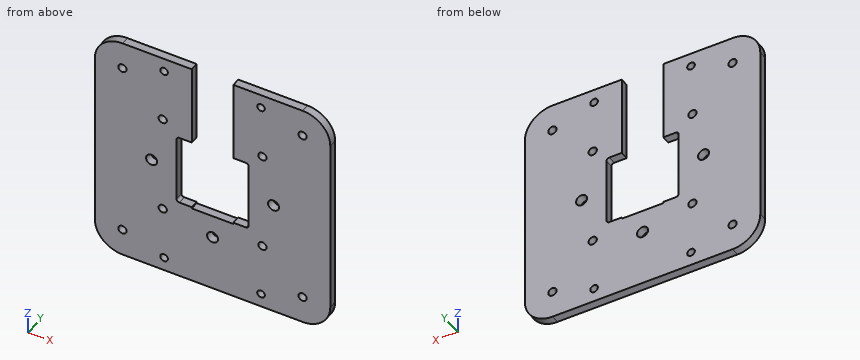
```python
from build123d import *

# Parameters (mm, degrees)
BOSS_EXTRUDE1_DEPTH = 3
FILLET1_R           = 10
CUT_EXTRUDE1_REACH  = 5
SKETCH2_R           = 1.5
SKETCH2_R_2         = 1.375
SKETCH2_R_3         = 2
CUT_EXTRUDE2_REACH  = 5
FILLET2_R           = 1


with BuildPart() as part:
    # Sketch1 → Boss-Extrude1 (new body)
    with BuildSketch(Plane(origin=(0, 0, 0), x_dir=(1, 0, 0), z_dir=(0, 1, 0))):
        Polygon((-42.5, -42.5), (42.5, -42.5), (42.5, -25), (42.5, 25), (42.5, 42.5), (-42.5, 42.5), align=None)
    extrude(amount=BOSS_EXTRUDE1_DEPTH)

    # Fillet1
    fillet1_edges = [part.edges().sort_by_distance(p)[0] for p in [
        (42.5, 1.5, 42.5),
        (-42.5, 1.5, 42.5),
        (-42.5, 1.5, -42.5),
        (42.5, 1.5, -42.5),
    ]]
    fillet(fillet1_edges, radius=FILLET1_R)

    # Sketch2 → Cut-Extrude1 (cut, up to next)
    with BuildSketch(Plane(origin=(0, 3, 0), x_dir=(1, 0, 0), z_dir=(0, 1, 0)), mode=Mode.PRIVATE) as cut_extrude1_sk1:
        with Locations((-32.5, 32.5)):
            Circle(SKETCH2_R)
    cut_extrude1_tool1 = extrude(cut_extrude1_sk1.sketch, amount=-CUT_EXTRUDE1_REACH, mode=Mode.PRIVATE) & part.part
    add(cut_extrude1_tool1.solids().sort_by_distance((-32.5, 3, -32.5))[0], mode=Mode.SUBTRACT)
    # Sketch2 → Cut-Extrude1 (cut, up to next)
    with BuildSketch(Plane(origin=(0, 3, 0), x_dir=(1, 0, 0), z_dir=(0, 1, 0)), mode=Mode.PRIVATE) as cut_extrude1_sk2:
        with Locations((32.5, 32.5)):
            Circle(SKETCH2_R)
    cut_extrude1_tool2 = extrude(cut_extrude1_sk2.sketch, amount=-CUT_EXTRUDE1_REACH, mode=Mode.PRIVATE) & part.part
    add(cut_extrude1_tool2.solids().sort_by_distance((32.5, 3, -32.5))[0], mode=Mode.SUBTRACT)
    # Sketch2 → Cut-Extrude1 (cut, up to next)
    with BuildSketch(Plane(origin=(0, 3, 0), x_dir=(1, 0, 0), z_dir=(0, 1, 0)), mode=Mode.PRIVATE) as cut_extrude1_sk3:
        with Locations((32.5, -32.5)):
            Circle(SKETCH2_R)
    cut_extrude1_tool3 = extrude(cut_extrude1_sk3.sketch, amount=-CUT_EXTRUDE1_REACH, mode=Mode.PRIVATE) & part.part
    add(cut_extrude1_tool3.solids().sort_by_distance((32.5, 3, 32.5))[0], mode=Mode.SUBTRACT)
    # Sketch2 → Cut-Extrude1 (cut, up to next)
    with BuildSketch(Plane(origin=(0, 3, 0), x_dir=(1, 0, 0), z_dir=(0, 1, 0)), mode=Mode.PRIVATE) as cut_extrude1_sk4:
        with Locations((-32.5, -32.5)):
            Circle(SKETCH2_R)
    cut_extrude1_tool4 = extrude(cut_extrude1_sk4.sketch, amount=-CUT_EXTRUDE1_REACH, mode=Mode.PRIVATE) & part.part
    add(cut_extrude1_tool4.solids().sort_by_distance((-32.5, 3, 32.5))[0], mode=Mode.SUBTRACT)
    # Sketch2 → Cut-Extrude1 (cut, up to next)
    with BuildSketch(Plane(origin=(0, 3, 0), x_dir=(1, 0, 0), z_dir=(0, 1, 0)), mode=Mode.PRIVATE) as cut_extrude1_sk5:
        with Locations((-17.5, -37.5)):
            Circle(SKETCH2_R_2)
    cut_extrude1_tool5 = extrude(cut_extrude1_sk5.sketch, amount=-CUT_EXTRUDE1_REACH, mode=Mode.PRIVATE) & part.part
    add(cut_extrude1_tool5.solids().sort_by_distance((-17.5, 3, 37.5))[0], mode=Mode.SUBTRACT)
    # Sketch2 → Cut-Extrude1 (cut, up to next)
    with BuildSketch(Plane(origin=(0, 3, 0), x_dir=(1, 0, 0), z_dir=(0, 1, 0)), mode=Mode.PRIVATE) as cut_extrude1_sk6:
        with Locations((17.5, -37.5)):
            Circle(SKETCH2_R_2)
    cut_extrude1_tool6 = extrude(cut_extrude1_sk6.sketch, amount=-CUT_EXTRUDE1_REACH, mode=Mode.PRIVATE) & part.part
    add(cut_extrude1_tool6.solids().sort_by_distance((17.5, 3, 37.5))[0], mode=Mode.SUBTRACT)
    # Sketch2 → Cut-Extrude1 (cut, up to next)
    with BuildSketch(Plane(origin=(0, 3, 0), x_dir=(1, 0, 0), z_dir=(0, 1, 0)), mode=Mode.PRIVATE) as cut_extrude1_sk7:
        with Locations((-18, 18)):
            Circle(SKETCH2_R)
    cut_extrude1_tool7 = extrude(cut_extrude1_sk7.sketch, amount=-CUT_EXTRUDE1_REACH, mode=Mode.PRIVATE) & part.part
    add(cut_extrude1_tool7.solids().sort_by_distance((-18, 3, -18))[0], mode=Mode.SUBTRACT)
    # Sketch2 → Cut-Extrude1 (cut, up to next)
    with BuildSketch(Plane(origin=(0, 3, 0), x_dir=(1, 0, 0), z_dir=(0, 1, 0)), mode=Mode.PRIVATE) as cut_extrude1_sk8:
        with Locations((-17.5, 37.5)):
            Circle(SKETCH2_R_2)
    cut_extrude1_tool8 = extrude(cut_extrude1_sk8.sketch, amount=-CUT_EXTRUDE1_REACH, mode=Mode.PRIVATE) & part.part
    add(cut_extrude1_tool8.solids().sort_by_distance((-17.5, 3, -37.5))[0], mode=Mode.SUBTRACT)
    # Sketch2 → Cut-Extrude1 (cut, up to next)
    with BuildSketch(Plane(origin=(0, 3, 0), x_dir=(1, 0, 0), z_dir=(0, 1, 0)), mode=Mode.PRIVATE) as cut_extrude1_sk9:
        with Locations((17.5, 37.5)):
            Circle(SKETCH2_R_2)
    cut_extrude1_tool9 = extrude(cut_extrude1_sk9.sketch, amount=-CUT_EXTRUDE1_REACH, mode=Mode.PRIVATE) & part.part
    add(cut_extrude1_tool9.solids().sort_by_distance((17.5, 3, -37.5))[0], mode=Mode.SUBTRACT)
    # Sketch2 → Cut-Extrude1 (cut, up to next)
    with BuildSketch(Plane(origin=(0, 3, 0), x_dir=(1, 0, 0), z_dir=(0, 1, 0)), mode=Mode.PRIVATE) as cut_extrude1_sk10:
        with Locations((18, 18)):
            Circle(SKETCH2_R)
    cut_extrude1_tool10 = extrude(cut_extrude1_sk10.sketch, amount=-CUT_EXTRUDE1_REACH, mode=Mode.PRIVATE) & part.part
    add(cut_extrude1_tool10.solids().sort_by_distance((18, 3, -18))[0], mode=Mode.SUBTRACT)
    # Sketch2 → Cut-Extrude1 (cut, up to next)
    with BuildSketch(Plane(origin=(0, 3, 0), x_dir=(1, 0, 0), z_dir=(0, 1, 0)), mode=Mode.PRIVATE) as cut_extrude1_sk11:
        with Locations((18, -18)):
            Circle(SKETCH2_R)
    cut_extrude1_tool11 = extrude(cut_extrude1_sk11.sketch, amount=-CUT_EXTRUDE1_REACH, mode=Mode.PRIVATE) & part.part
    add(cut_extrude1_tool11.solids().sort_by_distance((18, 3, 18))[0], mode=Mode.SUBTRACT)
    # Sketch2 → Cut-Extrude1 (cut, up to next)
    with BuildSketch(Plane(origin=(0, 3, 0), x_dir=(1, 0, 0), z_dir=(0, 1, 0)), mode=Mode.PRIVATE) as cut_extrude1_sk12:
        with Locations((-18, -18)):
            Circle(SKETCH2_R)
    cut_extrude1_tool12 = extrude(cut_extrude1_sk12.sketch, amount=-CUT_EXTRUDE1_REACH, mode=Mode.PRIVATE) & part.part
    add(cut_extrude1_tool12.solids().sort_by_distance((-18, 3, 18))[0], mode=Mode.SUBTRACT)
    # Sketch2 → Cut-Extrude1 (cut, up to next)
    with BuildSketch(Plane(origin=(0, 3, 0), x_dir=(1, 0, 0), z_dir=(0, 1, 0)), mode=Mode.PRIVATE) as cut_extrude1_sk13:
        with Locations((-22, 0)):
            Circle(SKETCH2_R_3)
    cut_extrude1_tool13 = extrude(cut_extrude1_sk13.sketch, amount=-CUT_EXTRUDE1_REACH, mode=Mode.PRIVATE) & part.part
    add(cut_extrude1_tool13.solids().sort_by_distance((-22, 3, 0))[0], mode=Mode.SUBTRACT)
    # Sketch2 → Cut-Extrude1 (cut, up to next)
    with BuildSketch(Plane(origin=(0, 3, 0), x_dir=(1, 0, 0), z_dir=(0, 1, 0)), mode=Mode.PRIVATE) as cut_extrude1_sk14:
        with Locations((0, 22)):
            Circle(SKETCH2_R_3)
    cut_extrude1_tool14 = extrude(cut_extrude1_sk14.sketch, amount=-CUT_EXTRUDE1_REACH, mode=Mode.PRIVATE) & part.part
    add(cut_extrude1_tool14.solids().sort_by_distance((0, 3, -22))[0], mode=Mode.SUBTRACT)
    # Sketch2 → Cut-Extrude1 (cut, up to next)
    with BuildSketch(Plane(origin=(0, 3, 0), x_dir=(1, 0, 0), z_dir=(0, 1, 0)), mode=Mode.PRIVATE) as cut_extrude1_sk15:
        with Locations((22, 0)):
            Circle(SKETCH2_R_3)
    cut_extrude1_tool15 = extrude(cut_extrude1_sk15.sketch, amount=-CUT_EXTRUDE1_REACH, mode=Mode.PRIVATE) & part.part
    add(cut_extrude1_tool15.solids().sort_by_distance((22, 3, 0))[0], mode=Mode.SUBTRACT)
    # Sketch2 → Cut-Extrude1 (cut, up to next)
    with BuildSketch(Plane(origin=(0, 3, 0), x_dir=(1, 0, 0), z_dir=(0, 1, 0)), mode=Mode.PRIVATE) as cut_extrude1_sk16:
        with Locations((0, -22)):
            Circle(SKETCH2_R_3)
    cut_extrude1_tool16 = extrude(cut_extrude1_sk16.sketch, amount=-CUT_EXTRUDE1_REACH, mode=Mode.PRIVATE) & part.part
    add(cut_extrude1_tool16.solids().sort_by_distance((0, 3, 22))[0], mode=Mode.SUBTRACT)

    # Sketch3 → Cut-Extrude2 (cut, up to next)
    with BuildSketch(Plane.XZ, mode=Mode.PRIVATE) as cut_extrude2_sk1:
        Polygon((7.5, -13.5), (-7.5, -13.5), (-7.5, -13), (-13, -13), (-13, 13), (-7.5, 13), (-7.5, 42.5), (7.5, 42.5), (7.5, 13), (13, 13), (13, -13), (7.5, -13), align=None)
    cut_extrude2_tool1 = extrude(cut_extrude2_sk1.sketch, amount=-CUT_EXTRUDE2_REACH, mode=Mode.PRIVATE) & part.part
    add(cut_extrude2_tool1.solids().sort_by_distance((0, 0, 10.817052))[0], mode=Mode.SUBTRACT)

    # Fillet2
    fillet2_edges = [part.edges().sort_by_distance(p)[0] for p in [
        (13, 1.5, 13),
        (13, 1.5, -13),
        (-13, 1.5, -13),
        (-13, 1.5, 13),
    ]]
    fillet(fillet2_edges, radius=FILLET2_R)


solid = part.part
```
Source: CAD feature listing. Evaluate the final solid. Frame: model axes, mm. Give positions to 0.01 mm unless a question says otherwise; leave off trailing zeros. Order: outer loops, then holes, each group sorted by start corner. A loop starts at its lowest first (then second) coordinate and runs counter-clockwise, first axis right, second up.
(1) Contact query for a flat-ended pin moving along its axis: P1, Ø1.5, axis at x = 0, y = 1, coming from the +Z side. Output: stop coordinate, or through.
(2) Material intervals for line 1 along Z through (x, y) = (-32.5, 1.8); line 2 along X through (y, z) = (1.75, -4); line 3 along X through (y, z) = (1.75, 18), sorted ascending.
(3) Section query A-A (x = 22). Return the cut outline in (y, z), plus the area to 3 significant figures.
(4) Section query C-C (z = -37.5). Return the cut outline in (x, y) (3 decimals).
(5) Section query B-B (z = 24.5). Return the cut outline in (x, y).
(6) Section query D-D (y = 1.1). State how many separate pieces and enclosed holes the cut face has, plus the area to 3 significant figures.
Outcome:
1. P1: stops at z = -13.5
2. line 1: z = -42.5 to -34, -31 to 31, 34 to 42.5
2. line 2: x = -42.5 to -13, 13 to 42.5
2. line 3: x = -42.5 to -19.5, -16.5 to -7.5, 7.5 to 16.5, 19.5 to 42.5
3. outline: (0, -42.5) - (3, -42.5) - (3, -2) - (0, -2) - close; (0, 2) - (3, 2) - (3, 42.5) - (0, 42.5) - close
3. area: 243 mm2
4. outline: (-41.16, 0) - (-18.875, 0) - (-18.875, 3) - (-41.16, 3) - close; (-16.125, 0) - (16.125, 0) - (16.125, 3) - (-16.125, 3) - close; (18.875, 0) - (41.16, 0) - (41.16, 3) - (18.875, 3) - close
5. outline: (-42.5, 0) - (-7.5, 0) - (-7.5, 3) - (-42.5, 3) - close; (7.5, 0) - (42.5, 0) - (42.5, 3) - (7.5, 3) - close
6. separate pieces: 1
6. enclosed holes: 15
6. area: 5,900 mm2
